For this review, use the dimensioned drawing (mm, ordinates from the lowest corner) and the shaded views. Round coordinates to 2 decimals unless told otherwise and drop trailing zeros. Write each loop counter-clockwise with the first axis right and the second up, starting at its lowest first coordinate (ties: lowest second). Pieces come first, ordered by that corner, then holes. Notation, with made-up numbers: (-34.75, 60) -> (6.25, 60) arc R18 ccw to (6.25, 64) -> close; hole circle Ø2 at (-31, -17.5). An arc over 180 degrees is marked (long way). Answer in a Markdown table with one row per item. Add a question column.
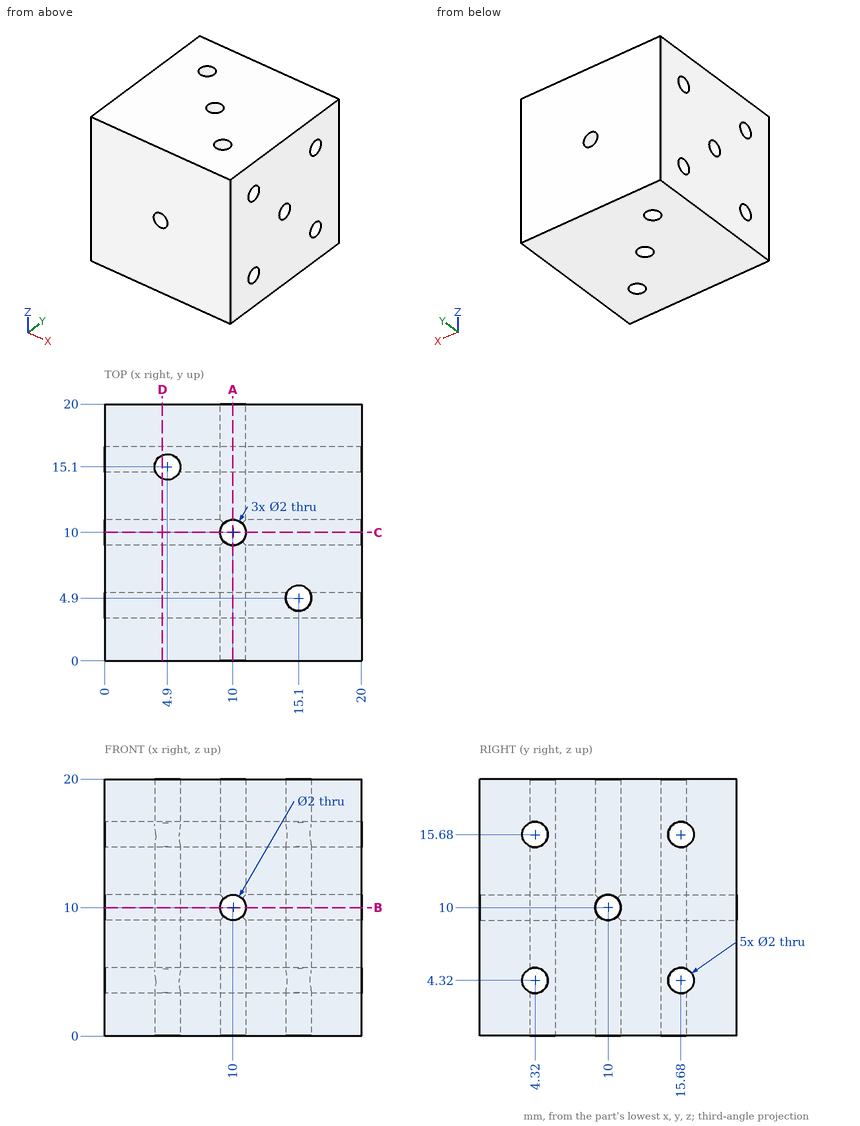
1. We need section C-C (y = 10). Write out the cut boundary in (x, z), plus the area to 3 significant figures.
2. We need section D-D (x = 4.5). Write out the cut boundary in (y, z), plus the area to 3 significant figures.
3. We need section B-B (z = 10). Write out the cut boundary in (x, y), plus the area to 3 significant figures.
4. Clearance check with a flat-ended pin moving along its axis: pin 1 Ø2.5 at (x, z) = (10, 10) entering from +Y. State where the tip first meets the part, or that it passes through.
5. We need section A-A (x = 10). Write out the cut boundary in (y, z).
6. For L1, parallel to Y at x = 15, z = 6 (1 decimal); L2, parallel to Y at x = 10, z = 6.5; L3, parallel to Z at x = 3.5, y = 16, list the stretches that pass through material, from the lowest coordinate up. Write a range as [from, to].
Response:
| question | item | result |
|---|---|---|
| 1 | outline | (0, 0) -> (9, 0) -> (9, 9) -> (0, 9) -> close; (0, 11) -> (9, 11) -> (9, 20) -> (0, 20) -> close; (11, 0) -> (20, 0) -> (20, 9) -> (11, 9) -> close; (11, 11) -> (20, 11) -> (20, 20) -> (11, 20) -> close |
| 1 | area | 324 mm2 |
| 2 | outline | (0, 0) -> (14.18, 0) -> (14.18, 20) -> (0, 20) -> close; (16.02, 0) -> (20, 0) -> (20, 20) -> (16.02, 20) -> (16.02, 16.62) arc R1 cw to (16.02, 14.74) -> (16.02, 5.26) arc R1 cw to (16.02, 3.38) -> close; hole circle Ø2 at (4.32, 4.32); hole circle Ø2 at (4.32, 15.68); hole circle Ø2 at (10, 10) |
| 2 | area | 352 mm2 |
| 3 | outline | (0, 0) -> (9, 0) -> (9, 9) -> (0, 9) -> close; (0, 11) -> (9, 11) -> (9, 20) -> (0, 20) -> close; (11, 0) -> (20, 0) -> (20, 9) -> (11, 9) -> close; (11, 11) -> (20, 11) -> (20, 20) -> (11, 20) -> close; hole circle Ø2 at (4.9, 15.1); hole circle Ø2 at (15.1, 4.9) |
| 3 | area | 318 mm2 |
| 4 | pin 1 | y = 20 |
| 5 | outline | (0, 0) -> (9, 0) -> (9, 9) -> (0, 9) -> close; (0, 11) -> (9, 11) -> (9, 20) -> (0, 20) -> close; (11, 0) -> (20, 0) -> (20, 9) -> (11, 9) -> close; (11, 11) -> (20, 11) -> (20, 20) -> (11, 20) -> close; hole circle Ø2 at (4.32, 4.32); hole circle Ø2 at (4.32, 15.68); hole circle Ø2 at (15.68, 4.32); hole circle Ø2 at (15.68, 15.68) |
| 6 | L1 | [0, 3.9], [5.9, 20] |
| 6 | L2 | [0, 9], [11, 20] |
| 6 | L3 | [0, 3.37], [5.27, 14.73], [16.63, 20] |
